Autodesk Inventor part; units mm, degrees
ref_plane "YZ Plane" through (0, 0, 0) normal (1, 0, 0) x (0, 1, 0)
ref_plane "XZ Plane" through (0, 0, 0) normal (0, 1, 0) x (-1, 0, 0)
ref_plane "XY Plane" through (0, 0, 0) normal (0, 0, 1) x (1, 0, 0)
sketch "Sketch1" plane through (0, 0, 0) normal (0, 0, 1) x (1, 0, 0)
  circle A0 centre (0, 0) radius 12.7
  arc A1 (50.8, 0) -> (-50.8, 0) centre (0, 0) ccw
  line L0 (-50.8, 0) -> (-50.8, -225.3234)
  line L1 (-50.8, -225.3234) -> (50.8, -225.3234)
  line L2 (50.8, -225.3234) -> (50.8, 0)
  circle A2 centre (176.5046, -179.1208) radius 32.385
  circle A3 centre (253.9746, -179.1208) radius 32.385
  line L3 (144.1196, -225.3234) -> (144.1196, -179.1208)
  line L4 (286.3596, -225.3234) -> (286.3596, -179.1208)
  line L5 (176.5046, -146.7358) -> (253.9746, -146.7358)
  line L6 (50.8, -225.3234) -> (144.1196, -225.3234)
  line L7 (286.3596, -225.3234) -> (508, -225.3234)
  line L8 (-50.8, -225.3234) -> (-238.2266, -225.3234)
  line L9 (-263.6266, -225.3234) -> (-263.6266, -150.876)
  line L10 (-263.6266, -150.876) -> (-212.8266, -150.876)
  line L11 (-212.8266, -150.876) -> (-212.8266, 50.8)
  line L12 (-212.8266, 50.8) -> (508, 50.8)
  line L13 (508, 50.8) -> (508, -225.3234)
  line L14 (-238.2266, -229.108) -> (-238.2266, -225.3234)
  line L15 (-238.2266, -229.108) -> (-263.6266, -229.108)
  line L16 (-263.6266, -229.108) -> (-263.6266, -225.3234)
  dimension "d0" = 176.5046
  dimension "d1" = 179.1208
  dimension "d2" = 64.77
  dimension "d3" = 64.77
  dimension "d4" = 77.47
  dimension "d5" = 212.8266
  dimension "d6" = 50.8
  dimension "d7" = 150.876
  dimension "d8" = 508
  dimension "d9" = 229.108
extrude "Extrusion1" add sketch "Sketch1" along normal blind 12.7 contours L2 L1 L0 A1 | A1 L12 L13 L7 L4 A3 L5 A2 L3 L6 L2 | A1 L0 L8 L14 L15 L16 L9 L10 L11 L12
sketch "Sketch2" plane through (0, 0, 0) normal (0, 0, -1) x (-1, 0, 0)
  line L0 (-286.3596, -225.3234) -> (-324.4596, -225.3234)
  line L1 (-324.4596, -225.3234) -> (-324.4596, -136.4234)
  line L2 (-324.4596, -136.4234) -> (-286.3596, -136.4234)
  line L3 (-286.3596, -136.4234) -> (-286.3596, -225.3234)
  line L4 (-144.1196, -225.3234) -> (-106.0196, -225.3234)
  line L5 (-106.0196, -225.3234) -> (-106.0196, -136.4234)
  line L6 (-106.0196, -136.4234) -> (-144.1196, -136.4234)
  line L7 (-144.1196, -136.4234) -> (-144.1196, -225.3234)
  dimension "d12" = 38.1
  dimension "d13" = 88.9
  dimension "d14" = 38.1
  dimension "d15" = 88.9
extrude "Extrusion2" add sketch "Sketch2" along normal blind 25.4
sketch "Sketch3" plane through (0, 0, -25.4) normal (0, 0, -1) x (-1, 0, 0)
  line L0 (-324.4596, -136.4234) -> (-106.0196, -136.4234)
  line L1 (-106.0196, -136.4234) -> (-106.0196, -225.3234)
  line L2 (-106.0196, -225.3234) -> (-324.4596, -225.3234)
  line L3 (-324.4596, -225.3234) -> (-324.4596, -136.4234)
  line L4 (-106.0196, -136.4234) -> (-106.0196, -225.3234)
  circle A0 centre (-225.1964, -177.5746) radius 12.7
  circle A1 centre (0, 0) radius 12.7
  dimension "d18" = 88.9
  dimension "d19" = 0
  dimension "d20" = 25.4
  dimension "d21" = 225.1964
extrude "Extrusion3" add sketch "Sketch3" along normal blind 12.7 contours L0 L1 L2 L3
sketch "Sketch4" plane through (0, 0, 12.7) normal (0, 0, 1) x (1, 0, 0)
  line L0 (286.3596, -225.3234) -> (508, -225.3234)
  line L1 (324.4596, -136.4234) -> (508, -60.2234)
  line L2 (508, -60.2234) -> (366.7969, -60.2234)
  arc A0 (508, -60.2234) -> (324.4596, -136.4234) centre (508, -319.3672) ccw
  line L3 (324.4596, -136.4234) -> (324.4596, -225.3234)
  line L4 (508, -60.2234) -> (324.4596, -60.2234)
  line L5 (324.4596, -60.2234) -> (324.4596, -225.3234)
  line L6 (324.4596, -225.3234) -> (508, -225.3234)
  line L7 (508, -225.3234) -> (508, -60.2234)
extrude "Extrusion4" cut sketch "Sketch4" against normal blind 25.4 contours L3 L1 L7 L0 | A0 L1
sketch "Sketch5" plane through (0, 0, -38.1) normal (0, 0, -1) x (-1, 0, 0)
  line L0 (-324.4596, -136.4234) -> (-324.4596, -225.3234)
  line L1 (-106.0196, -225.3234) -> (-106.0196, -136.4234)
  line L2 (-106.0196, -136.4234) -> (-324.4596, -136.4234)
  arc A0 (-235.5596, -136.4234) -> (-324.4596, -225.3234) centre (-235.5596, -225.3234) ccw
  line L3 (-324.4596, -225.3234) -> (-235.5596, -136.4234) construction
  line L4 (-324.4596, -225.3234) -> (-198.736, -225.3234) construction
  arc A1 (-106.0196, -225.3234) -> (-194.9196, -136.4234) centre (-194.9196, -225.3234) ccw
  line L5 (-106.0196, -225.3234) -> (-194.9196, -136.4234) construction
  line L6 (-106.0196, -225.3234) -> (19.704, -225.3234) construction
  point P0 (0, 0)
  dimension "d26" = 45
  dimension "d27" = 135
extrude "Extrusion5" cut sketch "Sketch5" against normal blind 38.1
fillet "Fillet1" radius 12.7 3 edges at (215.2396, -136.4234, -38.1) (132.0578, -162.4616, -38.1) (298.4214, -162.4616, -38.1)
sketch "Sketch6" plane through (0, 0, 12.7) normal (0, 0, 1) x (1, 0, 0)
  arc A0 (508, -60.2234) -> (324.4596, -136.4234) centre (508, -319.3672) ccw
  line L0 (508, -60.2234) -> (508, 50.8)
  line L1 (508, 50.8) -> (-212.8266, 50.8)
  line L2 (-212.8266, 50.8) -> (-212.8266, -150.876)
  line L3 (-212.8266, -150.876) -> (-263.6266, -150.876)
  line L4 (-263.6266, -150.876) -> (-263.6266, -229.108)
  line L5 (-263.6266, -229.108) -> (-238.2266, -229.108)
  line L6 (-238.2266, -229.108) -> (-238.2266, -225.3234)
  line L7 (-238.2266, -225.3234) -> (144.1196, -225.3234)
  line L8 (144.1196, -225.3234) -> (144.1196, -179.1208)
  arc A1 (176.5046, -146.7358) -> (144.1196, -179.1208) centre (176.5046, -179.1208) ccw
  line L9 (176.5046, -146.7358) -> (253.9746, -146.7358)
  arc A2 (286.3596, -179.1208) -> (253.9746, -146.7358) centre (253.9746, -179.1208) ccw
  line L10 (286.3596, -179.1208) -> (286.3596, -225.3234)
  line L11 (286.3596, -225.3234) -> (324.4596, -225.3234)
  line L12 (324.4596, -225.3234) -> (324.4596, -136.4234)
  circle A3 centre (0, 0) radius 12.7
sketch "Sketch7" plane through (0, 0, 12.7) normal (0, 0, 1) x (1, 0, 0)
  line L0 (324.4596, -225.3234) -> (324.4596, -136.4234)
  circle A0 centre (0, 0) radius 12.7
  line L1 (12.7, 0) -> (283.972, 0)
  circle A1 centre (283.972, 0) radius 35.56
  dimension "d31" = 271.272
  dimension "d32" = 71.12
extrude "Extrusion6" cut sketch "Sketch7" against normal blind 25.4 contours A1
properties part number "Shooter_TopMotorSupportRight"
Source: CAD feature listing. Evaluate the final solid. Frame: model axes, mm. A direction names the side the tool comes from. Round coordinates to 2 decimals unless told otherwise and drop trailing zeros. Loops run counter-clockwise (first coordinate to the right, second up) from the corner with the lowest first, then second, coordinate; pieces in that order, holes last. Notation, with made-up numbers: (76.25, 74) -> (114.25, 74) arc R15 cw to (114.25, 99) -> close; hole circle Ø10 at (25.5, 0.5). An arc over 180 degrees is marked (long way). Answer as a JSON object with one key per item and string values. Group by question number.
Q1. Section query B-B (y = 0). Output: boundary loops of the cut face in (x, z), plus the area to 3 significant figures.
Q2. Mould query, pull axis Z, two halves, no side actions, for faces 4 (the cylindrical face through (257.76, 24.03, 6.44)), 5 (the flat face through (144.12, -189, -7)), 6 (the flat face through (117, -87, 12.7)). Classes: pulls with the +Z half, pulls with the -Z half, needs draft (parallel to the pull), parting line crosses it, or undercut.
Q3. Ray query, line 1 (X direction, y = -179.5, z = -26.5); line 2 (Z direction, x = 328, y = -10); line 3 (Y direction, x = 0, z = 4). Return the intervals inside material, ascending. Write a range as from..to.
Q4. Section query A-A (x = 0). Output: boundary loops of the cut face in (y, z).
Q5. Contact query for flat-ended pins moving along their axis: P1, Ø10, axis at y = -21, z = 8.5, coming from the -X side; P2, Ø1.5, axis at y = -177.5, z = 2.5, coming from the +X side; P3, Ø6.5, axis at x = 229.5, z = 8, coming from the -Y side. Output: stop coordinate, or through.
Q6. Access query for faces 1 (the flat face through (-239, -150.876, 6)), 2 (the cylindrical face through (315.712, -186.869, -12.878)), 3 (the cylindrical face through (121.54, -175.14, -12.88)). Directions: +Z, -Z, +X, -X, +Y, -Y. A direction counts if a zero-diameter tool reaches every point of the face in a straight line with its end or side. Return the directions, or none.
Q7. Section query C-C (y = -44.5). Output: boundary loops of the cut face in (x, z), plus the area to 3 significant figures.
Q8. Section query D-D (x = 437). Output: boundary loops of the cut face in (y, z).
Completed:
{
 "1": {"outline": "(-212.83, 0) -> (-12.7, 0) -> (-12.7, 12.7) -> (-212.83, 12.7) -> close; (12.7, 0) -> (248.41, 0) -> (248.41, 12.7) -> (12.7, 12.7) -> close; (319.53, 0) -> (508, 0) -> (508, 12.7) -> (319.53, 12.7) -> close", "area": "7,930 mm²"},
 "2": {"face 4": "needs draft", "face 5": "undercut", "face 6": "pulls with the +Z half"},
 "3": {"line 1": "118.8..212.64, 237.75..311.68", "line 2": "0..12.7", "line 3": "-225.32..-12.7, 12.7..50.8"},
 "4": {"outline": "(-225.32, 0) -> (-12.7, 0) -> (-12.7, 12.7) -> (-225.32, 12.7) -> close; (12.7, 0) -> (50.8, 0) -> (50.8, 12.7) -> (12.7, 12.7) -> close"},
 "5": {"P1": "x = -212.83", "P2": "x = 324.46", "P3": "y = -146.74"},
 "6": {"face 1": "+Z, -Z, -X, +Y", "face 2": "-Z, +X, +Y", "face 3": "-Z, -X, +Y"},
 "7": {"outline": "(-212.83, 0) -> (508, 0) -> (508, 12.7) -> (-212.83, 12.7) -> close", "area": "9,150 mm²"},
 "8": {"outline": "(-70.14, 0) -> (50.8, 0) -> (50.8, 12.7) -> (-70.14, 12.7) -> close"}
}
